Here's how the part is built. I have some questions about the finished solid (model axes, mm). Coordinates: 2 decimals unless noted, no trailing zeros. Answer as CSV lines item,"result". Start each with the question number.
Item 1: I need wall thicknesses on line 1 (Z direction, x = 102, y = 0.55); line 2 (X direction, y = 0.2, z = -56.5); line 3 (Z direction, x = 104.26, y = 1.05). Which ranges of each line are inside material? Lowest first, please.
Item 2: Imagine slicing it at A-A on y = 0.35. Count the separate pieces of the cut face and the enclosed holes in it, and give its area (3 significant figures).
Item 3: We'd pull the mould along X, two halves only. Please class faces 1 (the face through (-114.4, 0.8, -58.8)), 2 (the face through (-13, 0, -125)): pulls with the +X half, pulls with the -X half, needs draft (parallel to the pull), parting line crosses it, or undercut.
Item 4: I'm going to push a flat-ended pin straight in: pin 1 (12 mm diameter, centred on x = -76.5, z = -127.5, fed in from -Y). Where does the tip first touch, or does it pass through?
from build123d import *

# Parameters (mm, degrees)
BOSS_EXTRU_1_DEPTH      = 1.5
ESQUISSE4_R             = 4
ESQUISSE4_R_2           = 1.5
ESQUISSE4_W             = 168
ESQUISSE4_H             = 102
ENL_V_MAT_EXTRU_3_DEPTH = 3
ENL_V_MAT_EXTRU_4_DEPTH = 1.5
ESQUISSE11_R            = 1.5
ENL_V_MAT_EXTRU_5_DEPTH = 1.5
CONG_1_R                = 1
ESQUISSE12_R            = 1.5
ENL_V_MAT_EXTRU_6_DEPTH = 224.924001117


# Read off the part's stored shape, not the designer's step: Enlèv. mat.-Extru.4
with BuildPart() as part:
    # Esquisse1 → Boss.-Extru.1 (new body)
    with BuildSketch(Plane(origin=(0, 0, 0), x_dir=(1, 0, 0), z_dir=(0, 1, 0))):
        with BuildLine():
            Line((-165, 6.391802297), (-165, 0))
            Line((-165, 0), (165, 0))
            Line((165, 0), (165, 6.391802297))
            add(Edge.make_bspline(
                [(165, 6.391802297), (0, 608.094924715), (-165, 6.391802297)],
                knots=[1.893832827, 1.893832827, 1.893832827, 4.38935248, 4.38935248, 4.38935248], degree=2, weights=[1, 0.317447459, 1]))
        make_face()
    extrude(amount=BOSS_EXTRU_1_DEPTH)

    # Esquisse4 → Enlèv. mat.-Extru.3 (cut)
    with BuildSketch(Plane(origin=(0, 1.5, 0), x_dir=(1, 0, 0), z_dir=(0, 1, 0))):
        with Locations(Location((-117.74, 61, 0), (0, 0, 270))):
            Circle(ESQUISSE4_R)
        with Locations(Location((-112.919092927, 55.254666677, 0), (0, 0, 270))):
            Circle(ESQUISSE4_R_2)
        with Locations(Location((-122.560907073, 66.745333323, 0), (0, 0, 270))):
            Circle(ESQUISSE4_R_2)
        with Locations(Location((-101.74, 61, 0), (0, 0, 270))):
            Circle(ESQUISSE4_R_2)
        with Locations(Location((104.26, 61, 0), (0, 0, 270))):
            Circle(ESQUISSE4_R_2)
        with Locations((1.26, 59)):
            Rectangle(ESQUISSE4_W, ESQUISSE4_H)
    extrude(amount=-ENL_V_MAT_EXTRU_3_DEPTH, mode=Mode.SUBTRACT)

    # Enlèv. mat.-Extru.4 outline → Enlèv. mat.-Extru.4 (cut)
    with BuildSketch(Plane(origin=(0, 0, 0), x_dir=(1, 0, 0), z_dir=(0, 1, 0))):
        with BuildLine():
            add(Edge.make_bspline(
                [(131.492595534, 29.994209065), (131.937846155, 45.779047079), (119, 45.779047079), (106.062153845, 45.779047079), (106.507404466, 29.994209065)],
                knots=[1.536374944, 1.536374944, 1.536374944, 3.141592654, 3.141592654, 4.746810363, 4.746810363, 4.746810363], degree=2, weights=[1, 0.694832863, 1, 0.694832863, 1]))
            add(Edge.make_bspline(
                [(106.507404466, 29.994209065), (106.062153845, 14.209371052), (119, 14.209371052), (131.937846155, 14.209371052), (131.492595534, 29.994209065)],
                knots=[4.677967597, 4.677967597, 4.677967597, 6.283185307, 6.283185307, 7.888403017, 7.888403017, 7.888403017], degree=2, weights=[1, 0.694832863, 1, 0.694832863, 1]))
        make_face()
    extrude(amount=ENL_V_MAT_EXTRU_4_DEPTH, mode=Mode.SUBTRACT)

    # Esquisse11 → Enlèv. mat.-Extru.5 (cut)
    with BuildSketch(Plane(origin=(0, 1.5, 0), x_dir=(1, 0, 0), z_dir=(0, 1, 0))):
        with Locations(Location((103, 29.994209065, 0), (0, 0, 270))):
            Circle(ESQUISSE11_R)
        with Locations(Location((135, 29.994209065, 0), (0, 0, 90))):
            Circle(ESQUISSE11_R)
    extrude(amount=-ENL_V_MAT_EXTRU_5_DEPTH, mode=Mode.SUBTRACT)

    # Congé1
    cong_1_edges = [part.edges().sort_by_distance(p)[0] for p in [
        (-82.74, 0.75, -110),
        (-82.74, 0.75, -8),
        (85.26, 0.75, -8),
        (85.26, 0.75, -110),
        (165, 0.75, 0),
        (-165, 0.75, 0),
    ]]
    fillet(cong_1_edges, radius=CONG_1_R)

    # Esquisse12 → Enlèv. mat.-Extru.6 (cut, through all)
    with BuildSketch(Plane(origin=(0, 1.5, 0), x_dir=(1, 0, 0), z_dir=(0, 1, 0))):
        with Locations(Location((-156, 15, 0), (0, 0, 270))):
            Circle(ESQUISSE12_R)
        with Locations(Location((-76, 123, 0), (0, 0, 270))):
            Circle(ESQUISSE12_R)
        with Locations(Location((-25, 143, 0), (0, 0, 270))):
            Circle(ESQUISSE12_R)
        with Locations(Location((25, 143, 0), (0, 0, 270))):
            Circle(ESQUISSE12_R)
        with Locations(Location((76, 123, 0), (0, 0, 270))):
            Circle(ESQUISSE12_R)
        with Locations(Location((156, 15, 0), (0, 0, 270))):
            Circle(ESQUISSE12_R)
        with Locations(Location((-102, 6, 0), (0, 0, 270))):
            Circle(ESQUISSE12_R)
        with Locations(Location((102, 6, 0), (0, 0, 270))):
            Circle(ESQUISSE12_R)
        with Locations(Location((-118, 86, 0), (0, 0, 270))):
            Circle(ESQUISSE12_R)
        with Locations(Location((118, 86, 0), (0, 0, 270))):
            Circle(ESQUISSE12_R)
        with BuildLine():
            Line((-4, 0), (4, 0))
            ThreePointArc((4, 0), (0, 2.438447187), (-4, 0))
        make_face()
    extrude(amount=-ENL_V_MAT_EXTRU_6_DEPTH, mode=Mode.SUBTRACT)


solid = part.part
Responses:
1,line 1,"z = -111.05 to -31.11, -28.88 to -7.5, -4.5 to 0"
1,line 2,"x = -144.93 to -113.76, -112.08 to -82.74, 85.26 to 144.93"
1,line 3,"z = -109.02 to -62.5, -59.5 to -30.81, -29.18 to 0"
2,separate pieces,"1"
2,enclosed holes,"19"
2,area,"19,200 mm^2"
3,face 1,"undercut"
3,face 2,"needs draft"
4,pin 1,"stops at y = 0"
